from build123d import *

# Parameters (mm, degrees)
SKETCH1_R           = 23.335
SKETCH1_R_2         = 13.335
BOSS_EXTRUDE1_DEPTH = 4
SKETCH3_R           = 57.5
SKETCH3_R_2         = 13.335
BOSS_EXTRUDE2_DEPTH = 5
SKETCH4_R           = 56
SKETCH4_R_2         = 51
SKETCH4_R_3         = 50
SKETCH4_R_4         = 45
SKETCH4_R_5         = 44
SKETCH4_R_6         = 39
SKETCH4_R_7         = 38
SKETCH4_R_8         = 33
SKETCH4_R_9         = 32
SKETCH4_R_10        = 27
CUT_EXTRUDE2_DEPTH  = 1.5
SKETCH5_R           = 2.5
SKETCH2_R           = 1.625
CUT_EXTRUDE1_DEPTH  = 82.813813015
SKETCH6_R           = 0.75
CUT_EXTRUDE3_DEPTH  = 82.503067427
SKETCH7_R           = 3
CUT_EXTRUDE4_DEPTH  = 3


with BuildPart() as part:
    # Sketch1 → Boss-Extrude1 (new body)
    with BuildSketch(Plane(origin=(0, 0, 0), x_dir=(1, 0, 0), z_dir=(0, 1, 0))):
        with Locations(Location((0, 0, 0), (0, 0, 270))):
            Circle(SKETCH1_R)
        with Locations(Location((0, 0, 0), (0, 0, 270))):
            Circle(SKETCH1_R_2, mode=Mode.SUBTRACT)
    extrude(amount=BOSS_EXTRUDE1_DEPTH)

    # Sketch3 → Boss-Extrude2 (add)
    with BuildSketch(Plane.XZ):
        with Locations(Location((0, 0, 0), (0, 0, 270))):
            Circle(SKETCH3_R)
        with Locations(Location((0, 0, 0), (0, 0, 270))):
            Circle(SKETCH3_R_2, mode=Mode.SUBTRACT)
    extrude(amount=BOSS_EXTRUDE2_DEPTH)

    # Sketch4 → Cut-Extrude2 (cut)
    with BuildSketch(Plane(origin=(0, 0, 0), x_dir=(1, 0, 0), z_dir=(0, 1, 0))):
        with Locations(Location((0, 0, 0), (0, 0, 270))):
            Circle(SKETCH4_R)
        with Locations(Location((0, 0, 0), (0, 0, 270))):
            Circle(SKETCH4_R_2, mode=Mode.SUBTRACT)
        with Locations(Location((0, 0, 0), (0, 0, 270))):
            Circle(SKETCH4_R_3)
        with Locations(Location((0, 0, 0), (0, 0, 270))):
            Circle(SKETCH4_R_4, mode=Mode.SUBTRACT)
        with Locations(Location((0, 0, 0), (0, 0, 270))):
            Circle(SKETCH4_R_5)
        with Locations(Location((0, 0, 0), (0, 0, 270))):
            Circle(SKETCH4_R_6, mode=Mode.SUBTRACT)
        with Locations(Location((0, 0, 0), (0, 0, 270))):
            Circle(SKETCH4_R_7)
        with Locations(Location((0, 0, 0), (0, 0, 270))):
            Circle(SKETCH4_R_8, mode=Mode.SUBTRACT)
        with Locations(Location((0, 0, 0), (0, 0, 270))):
            Circle(SKETCH4_R_9)
        with Locations(Location((0, 0, 0), (0, 0, 270))):
            Circle(SKETCH4_R_10, mode=Mode.SUBTRACT)
    extrude(amount=-CUT_EXTRUDE2_DEPTH, mode=Mode.SUBTRACT)

    # Sketch5 → Cut-Revolve1 (revolve, cut)
    with BuildSketch(Plane.XY, mode=Mode.PRIVATE) as cut_revolve1_sk:
        with Locations((-23.335, 4)):
            Circle(SKETCH5_R)
    revolve(cut_revolve1_sk.sketch.rotate(Axis((0, 4, 0), (0, -1, 0)), 90), axis=Axis((0, 4, 0), (0, -1, 0)), mode=Mode.SUBTRACT)

    # Sketch2 → Cut-Extrude1 (cut, through all)
    with BuildSketch(Plane(origin=(0, 4, 0), x_dir=(1, 0, 0), z_dir=(0, 1, 0))):
        with Locations(Location((-8.5425, 14.796044024, 0), (0, 0, 270))):
            Circle(SKETCH2_R)
        with Locations(Location((-17.085, 0, 0), (0, 0, 270))):
            Circle(SKETCH2_R)
        with Locations(Location((-8.5425, -14.796044024, 0), (0, 0, 270))):
            Circle(SKETCH2_R)
        with Locations(Location((8.5425, -14.796044024, 0), (0, 0, 270))):
            Circle(SKETCH2_R)
        with Locations(Location((17.085, 0, 0), (0, 0, 270))):
            Circle(SKETCH2_R)
        with Locations(Location((8.5425, 14.796044024, 0), (0, 0, 270))):
            Circle(SKETCH2_R)
    extrude(amount=-CUT_EXTRUDE1_DEPTH, mode=Mode.SUBTRACT)

    # Sketch6 → Cut-Extrude3 (cut, through all)
    with BuildSketch(Plane(origin=(0, -1.5, 0), x_dir=(1, 0, 0), z_dir=(0, 1, 0))):
        with Locations(Location((-53.5, 0, 0), (0, 0, 270))):
            Circle(SKETCH6_R)
        with Locations(Location((-47.5, 0, 0), (0, 0, 270))):
            Circle(SKETCH6_R)
        with Locations(Location((-41.5, 0, 0), (0, 0, 270))):
            Circle(SKETCH6_R)
        with Locations(Location((-35.5, 0, 0), (0, 0, 270))):
            Circle(SKETCH6_R)
        with Locations(Location((-29.5, 0, 0), (0, 0, 270))):
            Circle(SKETCH6_R)
    extrude(amount=-CUT_EXTRUDE3_DEPTH, mode=Mode.SUBTRACT)

    # Sketch7 → Cut-Extrude4 (cut)
    with BuildSketch(Plane.XZ.offset(5)):
        with Locations(Location((-17.085, 0, 0), (0, 0, 270))):
            Circle(SKETCH7_R)
        with Locations(Location((8.5425, -14.796044024, 0), (0, 0, 270))):
            Circle(SKETCH7_R)
        with Locations(Location((8.5425, 14.796044024, 0), (0, 0, 270))):
            Circle(SKETCH7_R)
    extrude(amount=-CUT_EXTRUDE4_DEPTH, mode=Mode.SUBTRACT)


solid = part.part
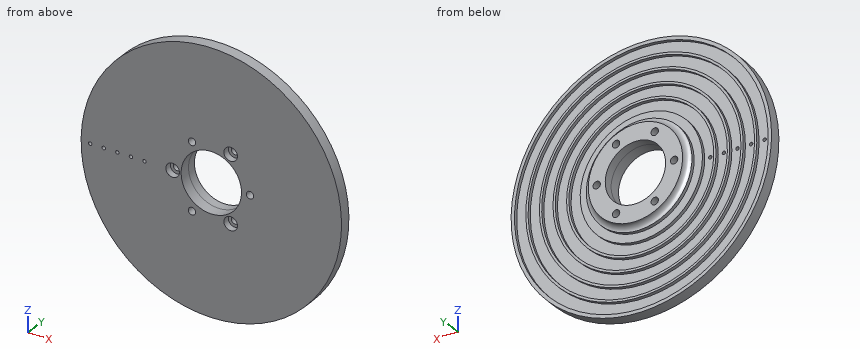
Here's how the part is built. I have some questions about the finished solid (model axes, mm). Give positions to 0.01 mm unless a question says otherwise; leave off trailing zeros. Order: outer loops, then holes, each group sorted by start corner. A loop starts at its lowest first (then second) coordinate and runs counter-clockwise, first axis right, second up. Notation, with made-up numbers: (53, 56) -> (101, 56) arc R13 cw to (101, 80) -> close; hole circle Ø7 at (61, 18.5). An arc over 180 degrees is marked (long way). Use a Markdown table: item, result. Add a question column.
Item 1: I need wall thicknesses on line 1 (Y direction, x = 49.5, z = 24.5); line 2 (X direction, y = -3.5, z = -37); line 3 (X direction, y = 0.25, z = -16). Which ranges of each line are inside material? Lowest first, please.
Item 2: Will these pins go through, and if not, where does the flat tip stop? pin 1 (1.5 mm diameter, centred on y = -2, z = 46, fed in from +X); pin 2 (1.5 mm diameter, centred on x = 5, y = -4, fed in from +Z); pin 3 (3 mm diameter, centred on y = 1, z = -26, fed in from +X).
Item 3: Imagine slicing it at A-A on z = 46.5. Please give me the cut outline in (x, y), plus the area to 3 significant figures.
Data:
| question | item | result |
|---|---|---|
| 1 | line 1 | y = -5 to -1.5 |
| 1 | line 2 | x = -44.01 to 44.01 |
| 1 | line 3 | x = -16.99 to -9.63, -7.45 to 7.45, 9.63 to 16.99 |
| 2 | pin 1 | stops at x = 35.48 |
| 2 | pin 2 | stops at z = 57.34 |
| 2 | pin 3 | stops at x = 51.84 |
| 3 | outline | (-33.82, -5) -> (33.82, -5) -> (33.82, 0) -> (31.2, 0) -> (31.2, -1.5) -> (20.95, -1.5) -> (20.95, 0) -> (18.38, 0) -> (18.38, -1.5) -> (-18.38, -1.5) -> (-18.38, 0) -> (-20.95, 0) -> (-20.95, -1.5) -> (-31.2, -1.5) -> (-31.2, 0) -> (-33.82, 0) -> close |
| 3 | area | 252 mm² |
